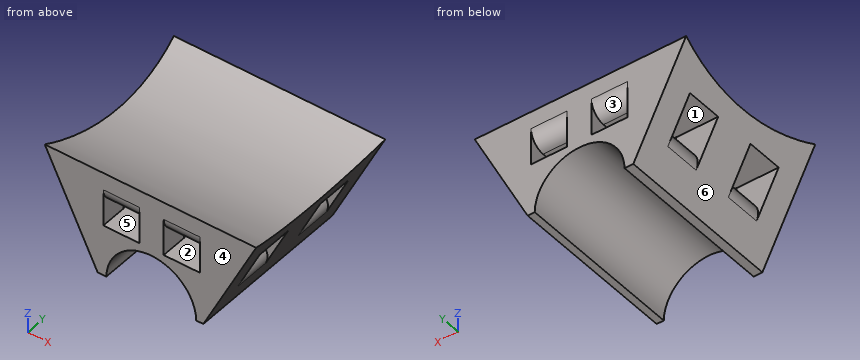
Autodesk Inventor part; units mm, degrees
ref_plane "YZ Plane" through (0, 0, 0) normal (1, 0, 0) x (0, 1, 0)
ref_plane "XZ Plane" through (0, 0, 0) normal (0, 1, 0) x (-1, 0, 0)
ref_plane "XY Plane" through (0, 0, 0) normal (0, 0, 1) x (1, 0, 0)
sketch "Sketch1" plane through (0, 0, 0) normal (1, 0, 0) x (0, 1, 0)
  line L0 (16, 10) -> (-16, 10)
  line L1 (-16, 10) -> (-16, -10)
  line L2 (-16, -10) -> (16, -10)
  line L3 (16, -10) -> (16, 10)
  line L4 (16, 10) -> (-16, -10) construction
  line L5 (-16, 10) -> (16, -10) construction
  point P0 (0, 0)
  dimension "d0" = 32
  dimension "d1" = 20
extrude "Extrusion1" add sketch "Sketch1" along normal blind 40
sketch "Sketch2" plane through (40, 0, 0) normal (1, 0, 0) x (0, 0, -1)
  line L0 (-10, 16) -> (-10, -16)
  line L1 (-10, 16) -> (-10, -16)
  arc A0 (-10, -16) -> (-10, 16) centre (-51.5241, 0) ccw
  point P0 (0, 0)
  dimension "d4" = 44.5
extrude "Extrusion2" cut sketch "Sketch2" against normal through all
sketch "Sketch3" plane through (0, 16, -10) normal (0, 1, 0) x (1, 0, 0)
  line L0 (11.6574, 0.0872) -> (28.6574, 0.0872)
  arc A0 (11.6574, 0.0872) -> (28.6574, 0.0872) centre (20.1574, 0.0872) ccw
  line L1 (0, -20) -> (0, 0)
  line L2 (10, 0) -> (0, -20)
  line L3 (0, -20) -> (0, 0)
  line L4 (0, 0) -> (10, 0)
  line L5 (40, 0) -> (40, -20)
  line L6 (30, 0) -> (40, -20)
  line L7 (40, -20) -> (40, 0)
  line L8 (30, 0) -> (40, 0)
  line L9 (0, 0) -> (40, 0)
  point P0 (0, -10)
  dimension "d8" = 17
  dimension "d36" = 10
  dimension "d37" = 10
extrude "Extrusion3" cut sketch "Sketch3" against normal through all
sketch "Sketch6" plane through (20.1574, 16, -10.0872) normal (0, 1, 0) x (1, 0, 0)
  line L0 (8.4996, -0.0872) -> (9.8426, -0.0872)
  line L1 (-9.0815, -13.7992) -> (-2.2244, -13.7992)
  line L2 (-2.2244, -13.7992) -> (-2.2244, -9.7992)
  line L3 (-2.2244, -9.7992) -> (-9.0815, -9.7992)
  line L4 (-9.0815, -9.7992) -> (-9.0815, -13.7992)
  line L5 (9.2042, -13.7992) -> (2.3471, -13.7992)
  line L6 (2.3471, -13.7992) -> (2.3471, -9.7992)
  line L7 (2.3471, -9.7992) -> (9.2042, -9.7992)
  line L8 (9.2042, -9.7992) -> (9.2042, -13.7992)
  point P0 (-20.1574, -10.0872)
  point P1 (-8.4996, -0.0872)
  dimension "d39" = 4
extrude "Extrusion4" cut sketch "Sketch6" against normal through all
fillet "Fillet3" radius 3 4 edges at (14.5045, -16, 3.7121) (25.933, -16, 3.7121) (14.5045, 16, 3.7121) (25.933, 16, 3.7121)
sketch "Sketch7" plane through (10, -16, -10) normal (-0.8944272, 0, -0.4472136) x (-0.4472136, 0, 0.8944272)
  line L0 (15.3752, 4.9726) -> (10.8752, 4.9726)
  line L1 (10.8752, 4.9726) -> (10.8752, 11.9726)
  line L2 (10.8752, 11.9726) -> (15.3752, 11.9726)
  line L3 (15.3752, 11.9726) -> (15.3752, 4.9726)
  line L4 (15.3752, 26.9631) -> (10.8752, 26.9631)
  line L5 (10.8752, 26.9631) -> (10.8752, 19.9631)
  line L6 (10.8752, 19.9631) -> (15.3752, 19.9631)
  line L7 (15.3752, 19.9631) -> (15.3752, 26.9631)
  point P0 (13.4164, 16)
  dimension "d40" = 4.5
  dimension "d41" = 7
  dimension "d43" = 7
sketch "Sketch8" plane through (0, -16, 10) normal (0, -1, 0) x (1, 0, 0)
  line L0 (-11.5037, -8.1401) -> (42.8743, -8.1401)
  line L1 (0, 0) -> (40, 0)
  point P0 (0, -10)
sweep "Sweep2" cut profiles "Sketch7" path "Sketch8" path curves L0
fillet "Fillet4" radius 3 4 edges at (5.1365, -7.5274, -0.2729) (5.1365, 7.4631, -0.2729) (34.8635, -7.5274, -0.2729) (34.8635, 7.4631, -0.2729)
properties part number "VHF_platform"
Work out the finished part from the listing and answer in its coordinate system (mm). Face numbers are marked on the shaded views. A direction names the side the tool comes from. Give positions to 0.01 mm unless a question says otherwise; leave off trailing zeros. Loops run counter-clockwise (first coordinate to the right, second up) from the corner with the lowest first, then second, coordinate; pieces in that order, holes last. Notation, with made-up numbers: (41.25, -28.5) -> (77.25, -28.5) arc R34 cw to (77.25, 3.5) -> close; hole circle Ø10 at (13, 82). An arc over 180 degrees is marked (long way). Use a Markdown table: item, result. Add a question column.
1. Section D-D on x = 20 is taken. Determine the outline of the cut face in (y, z).
2. For the marked faces 1, 2 and 3, determine the directions among +Z, -Z, +X, -X, +Y, -Y from which every point of the face is accessible in a straight line to the end or side of a thin tool.
3. Section B-B on z = 7.5 is taken. Determine the outline of the cut face in (x, y).
4. Flat-ended cylindrical pins translate along their axes: pin 1 Ø0.9 at (x, y) = (10.5, 8.5) entering from +Z; pin 2 Ø5.5 at (x, y) = (25, -7.5) entering from +Z; pin 3 Ø3.5 at (x, y) = (15.5, 2) entering from +Z. Find the tip coordinate at first contact, or state that the pin passes through.
5. Find the intervals of material crossed by probe 1 along Y at (x, z) = (32, 2.75); probe 2 along X at (y, z) = (-2.5, 1); probe 3 along X at (y, z) = (12.5, 0), in increasing order.
6. Section C-C on x = 34 is taken. Determine the outline of the cut face in (y, z), and give its area (3 significant figures).
7. Determine the mould class of the marked faces 4, 5 and 6 for opening direction X: released by +X, released by -X, zero draft, split by the parting line, or undercut.
Results below:
| question | item | result |
|---|---|---|
| 1 | outline | (-16, -1.59) -> (16, -1.59) -> (16, 10) arc R44.5 cw to (-16, 10) -> close; hole (-11.03, -0.27) -> (-4.03, -0.27) -> (-4.03, 3.75) -> (-11.03, 3.75) -> close; hole (3.96, -0.27) -> (10.96, -0.27) -> (10.96, 3.75) -> (3.96, 3.75) -> close |
| 2 | face 1 | +X, -X |
| 2 | face 2 | +Y, -Y |
| 2 | face 3 | +Y |
| 3 | outline | (1.25, -16) -> (38.75, -16) -> (38.75, -6.49) -> (1.25, -6.49) -> close; (1.25, 6.49) -> (38.75, 6.49) -> (38.75, 16) -> (1.25, 16) -> close |
| 4 | pin 1 | stops at z = 7.93 |
| 4 | pin 2 | stops at z = 8.22 |
| 4 | pin 3 | stops at z = 7.18 |
| 5 | probe 1 | y = -16 to -11.03, -4.03 to 3.96, 10.96 to 16 |
| 5 | probe 2 | x = 4.5 to 11.08, 17.93 to 22.5, 29.36 to 35.5 |
| 5 | probe 3 | x = 5 to 11.08, 17.93 to 22.5, 29.36 to 35 |
| 6 | outline | (-16, -2) -> (-11.03, -2) -> (-11.03, 3.75) -> (-4.03, 3.75) -> (-4.03, -2) -> (3.96, -2) -> (3.96, 3.75) -> (10.96, 3.75) -> (10.96, -2) -> (16, -2) -> (16, 10) arc R44.5 cw to (-16, 10) -> close |
| 6 | area | 240 mm^2 |
| 7 | face 4 | zero draft |
| 7 | face 5 | undercut |
| 7 | face 6 | released by -X |
